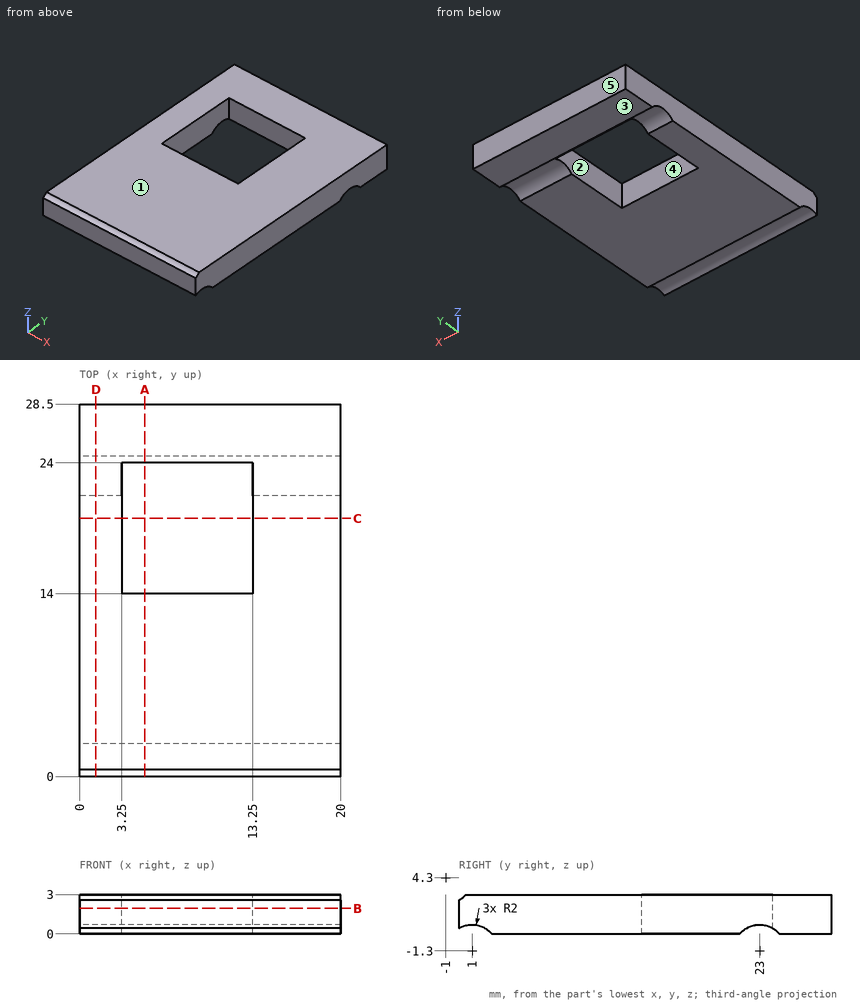
Drawing for the job (mm, zero at the part's lowest x, y, z). A direction names the side the tool comes from. Coordinates: 2 decimals unless noted, no trailing zeros. Order: outer loops, then holes, each group sorted by start corner. A loop starts at its lowest first (then second) coordinate and runs counter-clockwise, first axis right, second up. Notation, with made-up numbers: (47, 16) - (80, 16) arc R19 ccw to (80, 39) - close; hole circle Ø4 at (63, 40). An arc over 180 degrees is marked (long way). Use a Markdown table: item, result. Add a question column.
(1) Saw through at C-C (y = 19.75). Give the cut face in (x, z), then the cut area to 3 significant figures.
(2) Which spindle directions (+Z, -Z, +X, -X, +Y, -Y) get a long thin tool onto all of the face, cutting with end or side? Do the marked faces 1 and 2. Say none if no direction does.
(3) Saw through at A-A (x = 5). Give the cut face in (y, z), then the cut area to 3 significant figures.
(4) Drill centre lines: line 1 along X through (y, z) = (22.5, 1); line 2 along Y through (x, z) = (5.25, 1.3); line 3 along Y through (x, z) = (18.5, 2.75). Where is each one in solid material? Low to high. Write a range as [from, to].
(5) Saw through at D-D (x = 1.25). Give the cut face in (y, z), then the cut area to 3 significant figures.
(6) Saw through at B-B (z = 1.95). Give the cut face in (x, y).
(7) Pull direction Y, two halves, no side cores. Call the marked faces 3, 4 and 5: +Y half, -Y half, draft (parallel to the pull), parting line (faces both ways), or undercut.
Solved:
| question | item | result |
|---|---|---|
| 1 | outline | (0, 0) - (3.25, 0) - (3.25, 3) - (0, 3) - close; (13.25, 0) - (20, 0) - (20, 3) - (13.25, 3) - close |
| 1 | area | 30.0 mm² |
| 2 | face 1 | +Z, +X, -X, +Y, -Y |
| 2 | face 2 | +Z, -Z |
| 3 | outline | (0, 0.43) arc R2 cw to (2.52, 0) - (14, 0) - (14, 3) - (0.52, 3) arc R2 cw to (0, 2.57) - close; (24, 0.43) arc R2 cw to (24.52, 0) - (28.5, 0) - (28.5, 3) - (24, 3) - close |
| 3 | area | 53.9 mm² |
| 4 | line 1 | x = [0, 3.25], [13.25, 20] |
| 4 | line 2 | y = [0, 14], [24, 28.5] |
| 4 | line 3 | y = [0.26, 28.5] |
| 5 | outline | (0, 0.43) arc R2 cw to (2.52, 0) - (21.48, 0) arc R2 cw to (24.52, 0) - (28.5, 0) - (28.5, 3) - (0.52, 3) arc R2 cw to (0, 2.57) - close |
| 5 | area | 82.5 mm² |
| 6 | outline | (0, 0) - (20, 0) - (20, 28.5) - (0, 28.5) - close; hole (3.25, 14) - (13.25, 14) - (13.25, 24) - (3.25, 24) - close |
| 7 | face 3 | draft |
| 7 | face 4 | undercut |
| 7 | face 5 | +Y half |
